Check sheet for the drawn part. Datum: minimum x, y, z corner. Units: mm. A direction names the side the tool comes from. Round coordinates to 2 decimals unless told otherwise and drop trailing zeros. Loops run counter-clockwise (first coordinate to the right, second up) from the corner with the lowest first, then second, coordinate; pieces in that order, holes last.
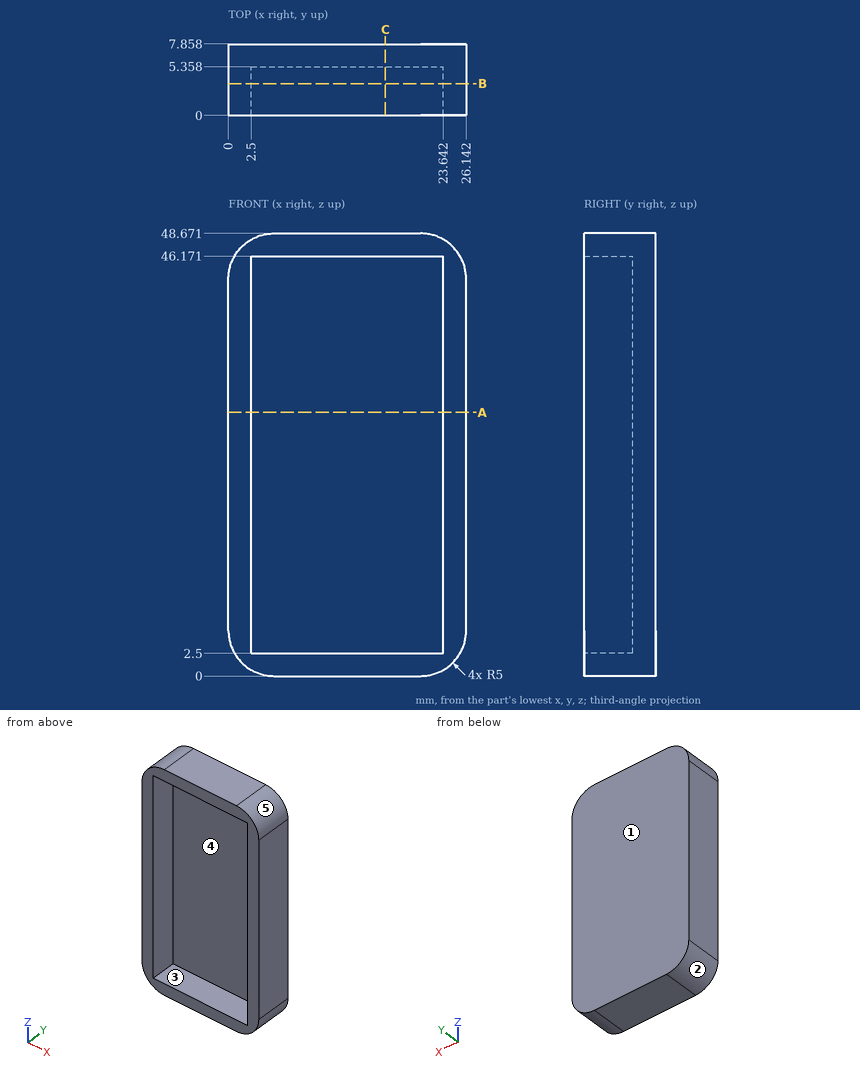
1) Access from +Z, -Z, +X, -X, +Y, -Y to the whole of each face (thin tool, end or side, straight path). Record for the marked faces 4 and 5.
Report:
face 4: -Y
face 5: +Z, +X, +Y, -Y
2) Sectioned sample at C-C, the plane x = 17.25. Record the cut outline in (y, z).
Report:
outline: (0, 0) - (7.86, 0) - (7.86, 48.67) - (0, 48.67) - (0, 46.17) - (5.36, 46.17) - (5.36, 2.5) - (0, 2.5) - close
3) Scan lines: line 1 along X through (y, z) = (5, 31); line 2 along Z through (x, y) = (16.75, 2); line 3 along Y through (x, z) = (23.5, 6.5). Record each from-to range of solid material in increasing order.
Report:
line 1: x = 0 to 2.5, 23.64 to 26.14
line 2: z = 0 to 2.5, 46.17 to 48.67
line 3: y = 5.36 to 7.86
4) Sectioned sample at B-B, the plane y = 3.5. Record the cut outline in (x, z).
Report:
outline: (0, 5) arc R5 ccw to (5, 0) - (21.14, 0) arc R5 ccw to (26.14, 5) - (26.14, 43.67) arc R5 ccw to (21.14, 48.67) - (5, 48.67) arc R5 ccw to (0, 43.67) - close; hole (2.5, 2.5) - (23.64, 2.5) - (23.64, 46.17) - (2.5, 46.17) - close
5) Mould release check, pull along X, two halves, no side actions. Record for the marked faces 1, 2 and 3: +X half, -X half, draft (parallel to the pull), parting line (faces both ways), or undercut.
Report:
face 1: draft
face 2: -X half
face 3: undercut
6) Sectioned sample at A-A, the plane z = 29. Record the cut outline in (x, y).
Report:
outline: (0, 0) - (2.5, 0) - (2.5, 5.36) - (23.64, 5.36) - (23.64, 0) - (26.14, 0) - (26.14, 7.86) - (0, 7.86) - close
7) Gauge pin test, flat ends, axial feed: pin 1 (1.5 mm diameter, centred on x = 8, z = 6.5, fed in from -Y); pin 2 (1.5 mm diameter, centred on y = 4, z = 6.5, fed in from -X). Record the tip position at first contact, or that the pin passes through.
Report:
pin 1: stops at y = 5.36
pin 2: stops at x = 0
